Input: part model. Units: mm. Frame: model coordinates. Face numbers are marked on the shaded views. A direction names the side the tool comes from. Coordinates: 2 decimals unless noted, no trailing zeros. Order: outer loops, then holes, each group sorted by start corner. A loop starts at its lowest first (then second) coordinate and runs counter-clockwise, first axis right, second up. Notation, with made-up numbers: (-20.75, 37.5) - (23.25, 37.5) arc R28 cw to (23.25, 57.5) - close; hole circle Ø9 at (86.5, 82.25). An arc over 180 degrees is marked (long way). Use a Markdown table: item, result. Add a question column.
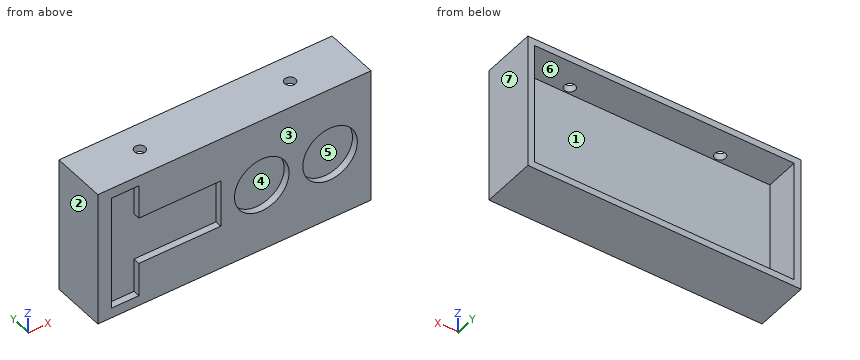
from build123d import *

# Parameters (mm, degrees)
F0_W     = 200
F0_H     = 100
F1_DEPTH = 40
F2_W     = 60
F2_H     = 35
F2_R     = 20
F3_DEPTH = 5
F4_W     = 190
F4_H     = 90
F5_DEPTH = 25
F6_R     = 4
F7_DEPTH = 40


with BuildPart() as f1:
    # F0 (on Front) → F1 (new body)
    with BuildSketch(Plane.XZ):
        Rectangle(F0_W, F0_H)
    extrude(amount=F1_DEPTH)

    # F2 (on face) → F3 (cut)
    with BuildSketch(Plane.XZ.offset(40)):
        Polygon((-90, -42.5), (-70, -42.5), (-70, -17.5), (-70, 17.5), (-70, 42.5), (-90, 42.5), align=None)
        with Locations((-40, 0)):
            Rectangle(F2_W, F2_H)
        with Locations((20, 0)):
            Circle(F2_R)
        with Locations((70, 0)):
            Circle(F2_R)
    extrude(amount=-F3_DEPTH, mode=Mode.SUBTRACT)

    # F4 (on face) → F5 (cut)
    with BuildSketch(Plane(origin=(0, 0, 0), x_dir=(-1, 0, 0), z_dir=(0, 1, 0))):
        Rectangle(F4_W, F4_H)
    extrude(amount=-F5_DEPTH, mode=Mode.SUBTRACT)

    # F6 (on face) → F7 (cut)
    with BuildSketch(Plane.XY.offset(50)):
        with Locations((-55, -20)):
            Circle(F6_R)
        with Locations((55, -20)):
            Circle(F6_R)
    extrude(amount=-F7_DEPTH, mode=Mode.SUBTRACT)


solid = f1.part
1) Cut plane A-A (y = -20). Return the cut outline in (x, z), and give its area (3 significant figures).
2) Pull-direction query (X, two-part tool) for the marked faces 1, 2, 3 and 4; classes: pulls with the +X half, pulls with the -X half, needs draft (parallel to the pull), parting line crosses it, or undercut.
3) Reachability of the marked faces 5, 6 and 7 from +Z, -Z, +X, -X, +Y, -Y: full face, straight path, thin tool, end or side. Return the list, or none.
4) Material intervals for L1, parallel to X at y = -10, z = 27; L2, parallel to Z at x = 88, y = -4.5; L3, parallel to Z at x = 70, y = -37, sorted ascending.
5) Cut plane D-D (x = 70). Return the cut outline in (y, z).
6) Cut plane B-B (x = -55). Return the cut outline in (y, z).
7) Contact query for flat-ended pins moving along their axis: P1, Ø2, axis at x = -28.5, z = -24, coming from the +Y side; P2, Ø12, axis at x = 67.5, z = 1.5, coming from the -Y side; P3, Ø24, axis at x = -59, z = 9.5, coming from the -Y side. Output: stop coordinate, or through.
8) Cut plane C-C (z = -32.5). Return the cut outline in (x, y).
Computed:
| question | item | result |
|---|---|---|
| 1 | outline | (-100, -50) - (100, -50) - (100, 50) - (59, 50) - (59, 45) - (95, 45) - (95, -45) - (-95, -45) - (-95, 45) - (-59, 45) - (-59, 50) - (-100, 50) - close; (-51, 45) - (51, 45) - (51, 50) - (-51, 50) - close |
| 1 | area | 2,820 mm2 |
| 2 | face 1 | undercut |
| 2 | face 2 | pulls with the -X half |
| 2 | face 3 | needs draft |
| 2 | face 4 | undercut |
| 3 | face 5 | -Y |
| 3 | face 6 | +Y |
| 3 | face 7 | +Z, -Z, +X, +Y, -Y |
| 4 | L1 | x = -100 to -95, 95 to 100 |
| 4 | L2 | z = -50 to -45, 45 to 50 |
| 4 | L3 | z = -50 to -20, 20 to 50 |
| 5 | outline | (-40, -50) - (0, -50) - (0, -45) - (-25, -45) - (-25, 45) - (0, 45) - (0, 50) - (-40, 50) - (-40, 20) - (-35, 20) - (-35, -20) - (-40, -20) - close |
| 6 | outline | (-40, -50) - (0, -50) - (0, -45) - (-25, -45) - (-25, 45) - (-24, 45) - (-24, 50) - (-40, 50) - (-40, 17.5) - (-35, 17.5) - (-35, -17.5) - (-40, -17.5) - close; (-16, 45) - (0, 45) - (0, 50) - (-16, 50) - close |
| 7 | P1 | stops at y = -25 |
| 7 | P2 | stops at y = -35 |
| 7 | P3 | stops at y = -40 |
| 8 | outline | (-100, -40) - (-90, -40) - (-90, -35) - (-70, -35) - (-70, -40) - (100, -40) - (100, 0) - (95, 0) - (95, -25) - (-95, -25) - (-95, 0) - (-100, 0) - close |
